Could you check a few things on this model? Use its own coordinates, in mm. A direction names the side the tool comes from. Round coordinates to 2 decimals unless told otherwise and drop trailing zeros. Loops run counter-clockwise (first coordinate to the right, second up) from the corner with the lowest first, then second, coordinate; pieces in that order, holes last. Notation, with made-up numbers: (35.5, 8) - (80.5, 8) arc R19 ccw to (80.5, 22) - close; hole circle Ø6 at (39.25, 60.5). An arc over 180 degrees is marked (long way). Use one line per item in the form item = value.
```python
from build123d import *

# Parameters (mm, degrees)
SKETCH1_R           = 10
BOSS_EXTRUDE1_DEPTH = 10
SKETCH2_R           = 10.638632356
SKETCH2_R_2         = 10
BOSS_EXTRUDE2_DEPTH = 10


with BuildPart() as part:
    # Sketch1 → Boss-Extrude1 (new body)
    with BuildSketch(Plane.XY):
        with BuildLine():
            Line((0, 15), (150, 15))
            ThreePointArc((150, 15), (165, 0), (150, -15))
            Line((150, -15), (0, -15))
            ThreePointArc((0, -15), (-15, 0), (0, 15))
        make_face()
        with Locations((75, 0)):
            Circle(SKETCH1_R, mode=Mode.SUBTRACT)
    extrude(amount=BOSS_EXTRUDE1_DEPTH)

    # Sketch2 → Boss-Extrude2 (add)
    with BuildSketch(Plane.XY.offset(10)):
        Circle(SKETCH2_R)
        with Locations((150, 0)):
            Circle(SKETCH2_R_2)
    extrude(amount=BOSS_EXTRUDE2_DEPTH)


solid = part.part
```
1. If we section it at A-A, the plane x = 75: Write out the boundary of the cut face in (y, z), plus the area to 3 significant figures.
Solution:
outline = (-15, 0) - (-10, 0) - (-10, 10) - (-15, 10) - close; (10, 0) - (15, 0) - (15, 10) - (10, 10) - close
area = 100 mm^2
2. If we section it at B-B, the plane z = 8.5: Write out the boundary of the cut face in (x, y), plus the area to 3 significant figures.
Solution:
outline = (0, -15) - (150, -15) arc R15 ccw to (150, 15) - (0, 15) arc R15 ccw to start; hole circle Ø20 at (75, 0)
area = 4,890 mm^2
3. On a 3-axis mill with a long thin cutter (end or side, diameter ignored), from which of +Z, -Z, +X, -X, +Y, -Y can I reach the whole of each face in a straight line? I mean faces 4 (the face through (159.237, -3.83, 14.93)), 5 (the face through (-15, 0, 5)). Say none if no direction works.
Solution:
face_4 = +Z
face_5 = +Z, -Z, -X
4. For P1, Ø1, axis at y = 7.5, z = 6, coming from the +X side; P2, Ø10, axis at y = 10, z = 13.5, coming from the +X side; P3, Ø12, axis at y = -7, z = 11, coming from the +X side; P4, Ø5, axis at y = 2.5, z = 2.5, coming from the -X side, each with a flat end and sliding along its axis, tell me the tip position at first contact or that it passes through.
Solution:
P1 = 163.27
P2 = 163.55
P3 = 164.96
P4 = -15
5. If we section it at C-C, the plane x = 147.5: Write out the boundary of the cut face in (y, z), plus the area to 3 significant figures.
Solution:
outline = (-15, 0) - (15, 0) - (15, 10) - (9.68, 10) - (9.68, 20) - (-9.68, 20) - (-9.68, 10) - (-15, 10) - close
area = 494 mm^2
6. Please list where these lines run through material, in increasing order: line 1 along Y through (x, z) = (75, 4); line 2 along Z through (x, y) = (144, -10.5); line 3 along X through (y, z) = (-9, 6.75).
Solution:
line_1 = -15 to -10, 10 to 15
line_2 = 0 to 10
line_3 = -12 to 70.64, 79.36 to 162
7. We'd pull the mould along Y, two halves only. Please class faces 1 (the face through (10.147, 3.196, 14.93)), 2 (the face through (65, 0, 5)), 3 (the face through (76.3, 10.2, 10)): +Y half, -Y half, draft (parallel to the pull), parting line (faces both ways), or undercut.
Solution:
face_1 = parting line
face_2 = undercut
face_3 = draft
